Verification items for the finished model (mm, model axes). A direction names the side the tool comes from. Give positions to 0.01 mm unless a question says otherwise; leave off trailing zeros. Order: outer loops, then holes, each group sorted by start corner. A loop starts at its lowest first (then second) coordinate and runs counter-clockwise, first axis right, second up. Notation, with made-up numbers: (10, -32) - (36, -32) arc R13 ccw to (36, -25) - close; hole circle Ø2 at (45, 52.25). An arc over 180 degrees is marked (long way). Answer as a JSON object with one key per item and string values.
```python
from build123d import *

# Parameters (mm, degrees)
BOSS_EXTRU_2_DEPTH       = 102.5
ESQUISSE7_R              = 1.75
ENL_V_MAT_EXTRU_4_DEPTH  = 12
ENL_V_START              = -5.6
ENL_V_MAT_EXTRU_5_DEPTH  = 2.6
ENL_V_START_2            = -12
ESQUISSE12_R             = 1.75
ENL_V_MAT_EXTRU_6_DEPTH  = 12
ENL_V_START_3            = -3
ENL_V_MAT_EXTRU_7_DEPTH  = 2.6
ENL_V_START_4            = -21
ESQUISSE18_W             = 14.3
ESQUISSE18_H             = 4.7
ENL_V_MAT_EXTRU_11_DEPTH = 11.74
ESQUISSE19_R             = 3.5
ENL_V_MAT_EXTRU_12_DEPTH = 105.622846453
ENL_V_START_5            = -2.5
ESQUISSE20_R             = 6.25
ENL_V_MAT_EXTRU_13_DEPTH = 103.122846576
ESQUISSE21_W             = 15
ESQUISSE21_H             = 15
ENL_V_MAT_EXTRU_14_DEPTH = 106.010713866
ESQUISSE22_W             = 2.25
ESQUISSE22_H             = 15.5
ENL_V_MAT_EXTRU_15_DEPTH = 9.125
CHANFREIN1_SIZE          = 9.125
CONG_1_R                 = 4
ESQUISSE23_W             = 6.93763889
ESQUISSE23_H             = 46
ENL_V_MAT_EXTRU_16_DEPTH = 106.010713866
CONG_2_R                 = 2


with BuildPart() as part:
    # Esquisse3 → Boss.-Extru.2 (new body)
    with BuildSketch(Plane.XY):
        with BuildLine():
            ThreePointArc((-20, 31.721443851), (0, 37.5), (20, 31.721443851))
            Line((20, 31.721443851), (14.06236111, 26.5))
            Line((14.06236111, 26.5), (-14.06236111, 26.5))
            Line((-14.06236111, 26.5), (-20, 31.721443851))
        make_face()
    extrude(amount=BOSS_EXTRU_2_DEPTH)

    # Esquisse7 → Enlèv. mat.-Extru.4 (cut)
    with BuildSketch(Plane.XY.offset(102.5)):
        with Locations((-12.915565842, 31.180934222)):
            Circle(ESQUISSE7_R)
        with Locations((12.915565842, 31.180934222)):
            Circle(ESQUISSE7_R)
    extrude(amount=-ENL_V_MAT_EXTRU_4_DEPTH, mode=Mode.SUBTRACT)

    # Esquisse11 → Enlèv. mat.-Extru.5 (cut)
    with BuildSketch(Plane.XY.offset(102.5).offset(ENL_V_START)):
        with BuildLine():
            Line((-15.765565842, 31.180934222), (-15.765565842, 34.024945756))
            ThreePointArc((-15.765565842, 34.024945756), (-12.95813326, 35.190009696), (-10.065565842, 36.123875543))
            Line((-10.065565842, 36.123875543), (-10.065565842, 29.426382489))
            Line((-10.065565842, 29.426382489), (-12.915565842, 27.780934222))
            Line((-12.915565842, 27.780934222), (-15.765565842, 29.426382489))
            Line((-15.765565842, 29.426382489), (-15.765565842, 31.180934222))
        make_face()
        with BuildLine():
            Line((10.065565842, 36.123875543), (10.065565842, 29.426382489))
            Line((10.065565842, 29.426382489), (12.915565842, 27.780934222))
            Line((12.915565842, 27.780934222), (15.765565842, 29.426382489))
            Line((15.765565842, 29.426382489), (15.765565842, 34.024945756))
            ThreePointArc((15.765565842, 34.024945756), (12.95813326, 35.190009696), (10.065565842, 36.123875543))
        make_face()
    extrude(amount=ENL_V_MAT_EXTRU_5_DEPTH, mode=Mode.SUBTRACT)

    # Esquisse12 → Enlèv. mat.-Extru.6 (cut)
    with BuildSketch(Plane(origin=(0, 0, 0), x_dir=(-1, 0, 0), z_dir=(0, 0, -1)).offset(ENL_V_START_2)):
        with Locations(Location((-12.915565842, 31.180934222, 0), (0, 0, 180))):
            Circle(ESQUISSE12_R)
        with Locations(Location((12.915565842, 31.180934222, 0), (0, 0, 180))):
            Circle(ESQUISSE12_R)
    extrude(amount=ENL_V_MAT_EXTRU_6_DEPTH, mode=Mode.SUBTRACT)

    # Esquisse14 → Enlèv. mat.-Extru.7 (cut)
    with BuildSketch(Plane(origin=(0, 0, 0), x_dir=(-1, 0, 0), z_dir=(0, 0, -1)).offset(ENL_V_START_3)):
        with BuildLine():
            Line((-15.765565842, 31.180934222), (-15.765565842, 34.024945756))
            ThreePointArc((-15.765565842, 34.024945756), (-12.95813326, 35.190009696), (-10.065565842, 36.123875543))
            Line((-10.065565842, 36.123875543), (-10.065565842, 29.426382489))
            Line((-10.065565842, 29.426382489), (-12.915565842, 27.780934222))
            Line((-12.915565842, 27.780934222), (-15.765565842, 29.426382489))
            Line((-15.765565842, 29.426382489), (-15.765565842, 31.180934222))
        make_face()
        with BuildLine():
            Line((10.065565842, 36.123875543), (10.065565842, 29.426382489))
            Line((10.065565842, 29.426382489), (12.915565842, 27.780934222))
            Line((12.915565842, 27.780934222), (15.765565842, 29.426382489))
            Line((15.765565842, 29.426382489), (15.765565842, 34.024945756))
            ThreePointArc((15.765565842, 34.024945756), (12.95813326, 35.190009696), (10.065565842, 36.123875543))
        make_face()
    extrude(amount=-ENL_V_MAT_EXTRU_7_DEPTH, mode=Mode.SUBTRACT)

    # Esquisse18 → Enlèv. mat.-Extru.11 (cut)
    with BuildSketch(Plane(origin=(0, 0, 0), x_dir=(-1, 0, 0), z_dir=(0, 0, -1)).offset(ENL_V_START_4)):
        with Locations((0, 28.85)):
            Rectangle(ESQUISSE18_W, ESQUISSE18_H)
    extrude(amount=-ENL_V_MAT_EXTRU_11_DEPTH, mode=Mode.SUBTRACT)

    # Esquisse19 → Enlèv. mat.-Extru.12 (cut, through all)
    with BuildSketch(Plane(origin=(0, 31.2, 0), x_dir=(-1, 0, 0), z_dir=(0, -1, 0))):
        with Locations(Location((0, -26.82, 0), (0, 0, 90))):
            Circle(ESQUISSE19_R)
    extrude(amount=-ENL_V_MAT_EXTRU_12_DEPTH, mode=Mode.SUBTRACT)

    # Esquisse20 → Enlèv. mat.-Extru.13 (cut, through all)
    with BuildSketch(Plane(origin=(0, 31.2, 0), x_dir=(-1, 0, 0), z_dir=(0, -1, 0)).offset(ENL_V_START_5)):
        with Locations(Location((0, -26.82, 0), (0, 0, 90))):
            Circle(ESQUISSE20_R)
    extrude(amount=-ENL_V_MAT_EXTRU_13_DEPTH, mode=Mode.SUBTRACT)

    # Esquisse21 → Enlèv. mat.-Extru.14 (cut, through all)
    with BuildSketch(Plane.XZ.offset(-26.5)):
        with Locations((0, 95)):
            Rectangle(ESQUISSE21_W, ESQUISSE21_H)
        with Locations((0, 7.5)):
            Rectangle(ESQUISSE21_W, ESQUISSE21_H)
    extrude(amount=-ENL_V_MAT_EXTRU_14_DEPTH, mode=Mode.SUBTRACT)

    # Esquisse22 → Enlèv. mat.-Extru.15 (cut)
    with BuildSketch(Plane(origin=(0, 26.5, 0), x_dir=(-1, 0, 0), z_dir=(0, -1, 0))):
        with Locations((-9.45, -82.5)):
            Rectangle(ESQUISSE22_W, ESQUISSE22_H)
    extrude(amount=-ENL_V_MAT_EXTRU_15_DEPTH, mode=Mode.SUBTRACT)

    # Chanfrein1
    # the kernel refuses this chamfer: 9.125 mm, written as the material it adds along each edge
    with BuildSketch(Plane(origin=(8.325, 35.625, 90.25), x_dir=(0, -0.9996219169112966, 0.027495876610586712), z_dir=(1, 0, 0)), Plane(origin=(10.575, 35.625, 74.75), x_dir=(0, -0.9996219169112966, -0.027495876610586712), z_dir=(-1, 0, 0))) as chanfrein1_piece_1:
        Polygon((CHANFREIN1_SIZE * 0.999621916911, CHANFREIN1_SIZE * 0.0274958766106), (-CHANFREIN1_SIZE * 0.0274958766106, CHANFREIN1_SIZE * 0.999621916911), (0, 0), align=None)
    extrude(amount=2.25)

    # Congé1
    cong_1_edges = [part.edges().sort_by_distance(p)[0] for p in [
        (9.45, 34.25, 82.5),
    ]]
    fillet(cong_1_edges, radius=CONG_1_R)

    # Esquisse23 → Enlèv. mat.-Extru.16 (cut, through all)
    with BuildSketch(Plane(origin=(0, 26.5, 0), x_dir=(-1, 0, 0), z_dir=(0, -1, 0))):
        with Locations((16.531180555, -36)):
            Rectangle(ESQUISSE23_W, ESQUISSE23_H)
    extrude(amount=-ENL_V_MAT_EXTRU_16_DEPTH, mode=Mode.SUBTRACT)

    # Congé2
    cong_2_edges = [part.edges().sort_by_distance(p)[0] for p in [
        (-13.06236111, 30.825727028, 59),
        (-13.06236111, 30.825727028, 13),
    ]]
    fillet(cong_2_edges, radius=CONG_2_R)


solid = part.part
```
(1) Section check C-C (z = 62). Record the cut outline in (x, y).
Computed values:
{"outline": "(-20, 31.72) - (-14.06, 26.5) - (14.06, 26.5) - (20, 31.72) arc R37.5 ccw to start"}
(2) Access from +Z, -Z, +X, -X, +Y, -Y to the whole of each face (thin tool, end or side, straight path). Record for faces 4 (the flat face through (0, 32, 87.5)), 5 (the flat face through (-10.066, 33, 4)), 6 (the flat face through (-13, 31, 12)), 7 (the cylindrical face through (-12.108, 29.628, 101.021)).
Computed values:
{"face 4": "+Z, +Y, -Y", "face 5": "+Y", "face 6": "-Z", "face 7": "+Z"}
(3) Section check A-A (x = 0). Record the cut outline in (y, z).
Computed values:
{"outline": "(26.5, 15) - (37.5, 15) - (37.5, 20.57) - (33.7, 20.57) - (33.7, 23.32) - (31.2, 23.32) - (31.2, 21) - (26.5, 21) - close; (26.5, 32.74) - (31.2, 32.74) - (31.2, 30.32) - (33.7, 30.32) - (33.7, 33.07) - (37.5, 33.07) - (37.5, 87.5) - (26.5, 87.5) - close"}
(4) Section check B-B (z = 26.82). Record the cut outline in (x, y).
Computed values:
{"outline": "(-13.06, 26.5) - (-7.15, 26.5) - (-7.15, 31.2) - (-3.5, 31.2) - (-3.5, 33.7) - (-6.25, 33.7) - (-6.25, 36.98) arc R37.5 ccw to (-13.06, 35.15) - close; (3.5, 31.2) - (7.15, 31.2) - (7.15, 26.5) - (14.06, 26.5) - (20, 31.72) arc R37.5 ccw to (6.25, 36.98) - (6.25, 33.7) - (3.5, 33.7) - close"}
(5) Gauge pin test, flat ends, axial feed: pin 1 Ø8 at (x, z) = (0, 26.82) entering from +Y; pin 2 Ø4.5 at (y, z) = (30, 31) entering from -X; pin 3 Ø2 at (x, y) = (9, 33) entering from -Z; pin 4 Ø4 at (x, z) = (-8.5, 36) entering from +Y. Record the tip position at first contact, or that the pin passes through.
Computed values:
{"pin 1": "stops at y = 33.7", "pin 2": "stops at x = -13.06", "pin 3": "stops at z = 0", "pin 4": "stops at y = 36.93"}
(6) Material ranges on line 1 along Z through (x, y) = (4.5, 29.5); line 2 along Z through (x, y) = (3.5, 35); line 3 along Y through (x, z) = (14, 92.5), recorded low to high. Write a range as [from, to].
Computed values:
{"line 1": "z = [15, 21], [32.74, 87.5]", "line 2": "z = [15, 21.64], [32, 87.5]", "line 3": "y = [26.5, 29.81], [32.55, 34.79]"}
(7) Section check D-D (z = 16). Record the cut outline in (x, y), then the cut area to 3 significant figures.
Computed values:
{"outline": "(-13.06, 26.5) - (14.06, 26.5) - (20, 31.72) arc R37.5 ccw to (-13.06, 35.15) - close", "area": "301 mm²"}
(8) Release check for a two-part mould opening along Z. For faces 1 (the flat face through (0, 26.5, 51)), 2 (the flat face through (10.575, 29, 83)), 3 (the flat face through (13, 31, 90.5)) record: pulls with the +Z half, pulls with the -Z half, needs draft (parallel to the pull), parting line crosses it, or undercut.
Computed values:
{"face 1": "needs draft", "face 2": "undercut", "face 3": "pulls with the +Z half"}
